from build123d import *

# Parameters (mm, degrees)
ESQUISSE1_W        = 120
ESQUISSE1_H        = 100
ESQUISSE1_W_2      = 39
ESQUISSE1_H_2      = 60
ESQUISSE1_W_3      = 31
ESQUISSE1_W_4      = 50
ESQUISSE1_H_3      = 20
ESQUISSE1_R        = 1.8
ESQUISSE1_W_5      = 61
ESQUISSE1_H_4      = 10
BOSS_EXTRU_1_DEPTH = 3


with BuildPart() as part:
    # Esquisse1 → Boss.-Extru.1 (new body)
    # profile 1 of 5: a face of its own
    with BuildSketch(Plane.XY):
        with Locations((60, 50)):
            Rectangle(ESQUISSE1_W, ESQUISSE1_H)
        with Locations((80.5, 50)):
            Rectangle(ESQUISSE1_W_2, ESQUISSE1_H_2, mode=Mode.SUBTRACT)
        with Locations((35.5, 50)):
            Rectangle(ESQUISSE1_W_3, ESQUISSE1_H_2, mode=Mode.SUBTRACT)
    # profile 2 of 5: a face of its own
    with BuildSketch(Plane.XY):
        with Locations((95, -10)):
            Rectangle(ESQUISSE1_W_4, ESQUISSE1_H_3)
        with Locations((75, -10)):
            Circle(ESQUISSE1_R, mode=Mode.SUBTRACT)
        with Locations((115, -10)):
            Circle(ESQUISSE1_R, mode=Mode.SUBTRACT)
    # profile 3 of 5: a face of its own
    with BuildSketch(Plane.XY):
        with Locations((30.5, -5)):
            Rectangle(ESQUISSE1_W_5, ESQUISSE1_H_4)
        with Locations((20, -5)):
            Circle(ESQUISSE1_R, mode=Mode.SUBTRACT)
        with Locations((41, -5)):
            Circle(ESQUISSE1_R, mode=Mode.SUBTRACT)
    # profile 4 of 5: a face of its own
    with BuildSketch(Plane.XY):
        with Locations((30.5, 105)):
            Rectangle(ESQUISSE1_W_5, ESQUISSE1_H_4)
        with Locations((20, 105)):
            Circle(ESQUISSE1_R, mode=Mode.SUBTRACT)
        with Locations((41, 105)):
            Circle(ESQUISSE1_R, mode=Mode.SUBTRACT)
    # profile 5 of 5: a face of its own
    with BuildSketch(Plane.XY):
        with Locations((95, 110)):
            Rectangle(ESQUISSE1_W_4, ESQUISSE1_H_3)
        with Locations((75, 110)):
            Circle(ESQUISSE1_R, mode=Mode.SUBTRACT)
        with Locations((115, 110)):
            Circle(ESQUISSE1_R, mode=Mode.SUBTRACT)
    extrude(amount=BOSS_EXTRU_1_DEPTH)


solid = part.part
Can you work these out from the model? Positions are in its coordinate system, mm. A direction names the side the tool comes from. Coordinates: 2 decimals unless noted, no trailing zeros. Write each loop counter-clockwise with the first axis right and the second up, starting at its lowest first coordinate (ties: lowest second). Pieces come first, ordered by that corner, then holes.
Q1. Imagine slicing it at D-D, the plane x = 115. List the corners of the cut face in (y, z) for me, plus the area to 3 significant figures.
Results found:
outline: (-20, 0) - (-11.8, 0) - (-11.8, 3) - (-20, 3) - close; (-8.2, 0) - (108.2, 0) - (108.2, 3) - (-8.2, 3) - close; (111.8, 0) - (120, 0) - (120, 3) - (111.8, 3) - close
area: 398 mm2
Q2. Imagine slicing it at A-A, the plane y = 45.5. List the corners of the cut face in (x, z) for me, plus the area to 3 significant figures.
Results found:
outline: (0, 0) - (20, 0) - (20, 3) - (0, 3) - close; (51, 0) - (61, 0) - (61, 3) - (51, 3) - close; (100, 0) - (120, 0) - (120, 3) - (100, 3) - close
area: 150 mm2
Q3. For P1, Ø0.9, axis at x = 63.5, z = 1.5, coming from the -Y side; P2, Ø0.9, axis at x = 39, z = 1, coming from the -Y side; P3, Ø3, axis at x = 20, y = -5, coming from the +Z side, each with a flat end and sliding along its axis, tell me the tip position at first contact or that it passes through.
Results found:
P1: stops at y = 0
P2: stops at y = -10
P3: passes through
Q4. If we mould it in two halves opening along X, with no side actions, what happens to faces 4 (the face through (95, -20, 1)), 5 (the face through (35, 80, 1))? For each: +X half, -X half, draft (parallel to the pull), parting line (faces both ways), or undercut.
Results found:
face 4: draft
face 5: undercut
Q5. Imagine slicing it at B-B, the plane x = 41. List the corners of the cut face in (y, z) for me, plus the area to 3 significant figures.
Results found:
outline: (-10, 0) - (-6.8, 0) - (-6.8, 3) - (-10, 3) - close; (-3.2, 0) - (20, 0) - (20, 3) - (-3.2, 3) - close; (80, 0) - (103.2, 0) - (103.2, 3) - (80, 3) - close; (106.8, 0) - (110, 0) - (110, 3) - (106.8, 3) - close
area: 158 mm2
Q6. Please list where these lines run through material, in increasing order: L1, parallel to X at y = 73, z = 1.2; L2, parallel to Y at x = 41, z = 0.8; L3, parallel to Y at x = 115, z = 1.25.
Results found:
L1: x = 0 to 20, 51 to 61, 100 to 120
L2: y = -10 to -6.8, -3.2 to 20, 80 to 103.2, 106.8 to 110
L3: y = -20 to -11.8, -8.2 to 108.2, 111.8 to 120
Q7. Imagine slicing it at C-C, the plane z = 1.6. Count the separate pieces of the cut face and the enclosed holes in it, plus the area to 3 significant figures.
Results found:
separate pieces: 1
enclosed holes: 10
area: 10,900 mm2
Q8. Which directions (+Z, -Z, +X, -X, +Y, -Y) give clear straight access to the entire face, cutting with the end or side of a thin tool? Please do faces 1 (the face through (65, 0, 1)), 2 (the face through (70, 110, 1)), 3 (the face through (51, 50, 1)).
Results found:
face 1: +Z, -Z, -Y
face 2: +Z, -Z, +Y
face 3: +Z, -Z
